Source: CAD feature listing. Evaluate the final solid. Frame: model axes, mm. Give positions to 0.01 mm unless a question says otherwise; leave off trailing zeros. Order: outer loops, then holes, each group sorted by start corner. A loop starts at its lowest first (then second) coordinate and runs counter-clockwise, first axis right, second up. Notation, with made-up numbers: (0, 7.25) - (33, 7.25) arc R10 cw to (33, 14.25) - close; hole circle Ø1 at (-11, 75.25). An arc over 180 degrees is marked (long way). Use CSV: the item, a comma, the result in double quotes.
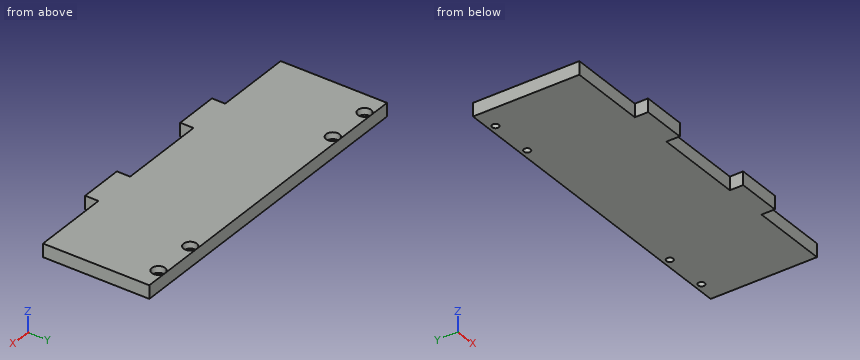
```python
from build123d import *

# Parameters (mm, degrees)
ESQUISSE1_W             = 150
ESQUISSE1_H             = 54
BOSS_EXTRU_1_DEPTH      = 6
ESQUISSE2_W             = 35
ESQUISSE2_H             = 6
ESQUISSE2_W_2           = 40
ENL_V_MAT_EXTRU_1_DEPTH = 160.536829604
ESQUISSE4_R             = 1.5
ENL_V_MAT_EXTRU_3_DEPTH = 6
ESQUISSE5_R             = 2.995
ENL_V_MAT_EXTRU_4_DEPTH = 3


with BuildPart() as part:
    # Esquisse1 → Boss.-Extru.1 (new body)
    with BuildSketch(Plane.XY):
        with Locations((-75, 27)):
            Rectangle(ESQUISSE1_W, ESQUISSE1_H)
    extrude(amount=BOSS_EXTRU_1_DEPTH)

    # Esquisse2 → Enlèv. mat.-Extru.1 (cut, through all)
    with BuildSketch(Plane.XY.offset(6)):
        with Locations((-17.5, 3)):
            Rectangle(ESQUISSE2_W, ESQUISSE2_H)
        with Locations((-75, 3)):
            Rectangle(ESQUISSE2_W_2, ESQUISSE2_H)
        with Locations((-132.5, 3)):
            Rectangle(ESQUISSE2_W, ESQUISSE2_H)
    extrude(amount=-ENL_V_MAT_EXTRU_1_DEPTH, mode=Mode.SUBTRACT)

    # Esquisse4 → Enlèv. mat.-Extru.3 (cut)
    with BuildSketch(Plane.XY.offset(6)):
        with Locations((-140, 51)):
            Circle(ESQUISSE4_R)
        with Locations((-120, 51)):
            Circle(ESQUISSE4_R)
        with Locations(Location((-30, 51, 0), (0, 0, 180))):
            Circle(ESQUISSE4_R)
        with Locations(Location((-10, 51, 0), (0, 0, 180))):
            Circle(ESQUISSE4_R)
    extrude(amount=-ENL_V_MAT_EXTRU_3_DEPTH, mode=Mode.SUBTRACT)

    # Esquisse5 → Enlèv. mat.-Extru.4 (cut)
    with BuildSketch(Plane.XY.offset(6)):
        with Locations((-140, 51)):
            Circle(ESQUISSE5_R)
        with Locations((-120, 51)):
            Circle(ESQUISSE5_R)
        with Locations(Location((-30, 51, 0), (0, 0, 180))):
            Circle(ESQUISSE5_R)
        with Locations(Location((-10, 51, 0), (0, 0, 180))):
            Circle(ESQUISSE5_R)
    extrude(amount=-ENL_V_MAT_EXTRU_4_DEPTH, mode=Mode.SUBTRACT)


solid = part.part
```
Item 1: Section A-A on z = 4.2. Return the cut outline in (x, y) (3 decimals), then the cut area to 3 significant figures.
Filled in:
outline,"(-150, 6) - (-115, 6) - (-115, 0) - (-95, 0) - (-95, 6) - (-55, 6) - (-55, 0) - (-35, 0) - (-35, 6) - (0, 6) - (0, 54) - (-150, 54) - close; hole circle Ø5.99 at (-140, 51); hole circle Ø5.99 at (-120, 51); hole circle Ø5.99 at (-30, 51); hole circle Ø5.99 at (-10, 51)"
area,"7,330 mm2"
Item 2: Section B-B on x = -120. Return the cut outline in (y, z) (3 decimals).
Filled in:
outline,"(6, 0) - (49.5, 0) - (49.5, 3) - (48.005, 3) - (48.005, 6) - (6, 6) - close; (52.5, 0) - (54, 0) - (54, 6) - (53.995, 6) - (53.995, 3) - (52.5, 3) - close"
Item 3: Material intervals for line 1 (Y direction, x = -10, z = 1.5); line 2 (X direction, y = 4.5, z = 5.7); line 3 (Y direction, x = -87, z = 5.05), sorted ascending. Write a range as from..to.
Filled in:
line 1,"y = 6..49.5, 52.5..54"
line 2,"x = -115..-95, -55..-35"
line 3,"y = 6..54"
Item 4: Section D-D on x = -74. Return the cut outline in (y, z).
Filled in:
outline,"(6, 0) - (54, 0) - (54, 6) - (6, 6) - close"
Item 5: Section C-C on y = 51. Count the separate pieces of the cut face and the enclosed holes in it, then the cut area to 3 significant figures.
Filled in:
separate pieces,"5"
enclosed holes,"0"
area,"792 mm2"
Item 6: First-contact query: pin 1 (3 mm diameter, centred on x = -11, y = 52, fed in from +Z); pin 2 (3 mm diameter, centred on x = -77, z = 2, fed in from -Y). Flat tips, straight axial feed; report the tip coordinate or a pass-through.
Filled in:
pin 1,"stops at z = 3"
pin 2,"stops at y = 6"
